```python
from build123d import *

# Parameters (mm, degrees)
SKETCH1_R             = 30
BOSS_EXTRUDE1_DEPTH   = 150
BOSS_EXTRUDE1_2_DEPTH = 150
EXTRUDE_THIN1_START   = -100
EXTRUDE_THIN1_DEPTH   = 100
SKETCH2_OUTSIDE_W     = 2224.156
SKETCH2_OUTSIDE_H     = 474.106
CUT_EXTRUDE1_DEPTH    = 100


# Read off the part's stored shape, not the designer's step: Extrude-Thin1
with BuildPart() as part:
    # Sketch1 → Boss-Extrude1 (new body)
    with BuildSketch(Plane(origin=(0, 0, 0), x_dir=(1, 0, 0), z_dir=(0, 1, 0))):
        with Locations(Location((0, 0, 0), (0, 0, 270))):
            Circle(SKETCH1_R)
    extrude(amount=-BOSS_EXTRUDE1_DEPTH)



with BuildPart() as body_2:
    # Sketch1 → Boss-Extrude1 2 (new body)
    with BuildSketch(Plane(origin=(0, 0, 0), x_dir=(1, 0, 0), z_dir=(0, 1, 0))):
        with Locations(Location((-1750.05, 0, 0), (0, 0, 270))):
            Circle(SKETCH1_R)
    extrude(amount=-BOSS_EXTRUDE1_2_DEPTH)


with BuildPart() as part_1:
    add(part.part)

    add(body_2.part)  # Extrude-Thin1 merges body 2
    # Extrude-Thin1 outline → Extrude-Thin1 (add)
    with BuildSketch(Plane.XY.offset(50).offset(EXTRUDE_THIN1_START)):
        with BuildLine():
            Line((-1500.05, -100), (-250, -100))
            add(Edge.make_bspline(
                [(-250, -100), (-180.532615563, -100), (-147.140452079, 0), (-100, 0)],
                knots=[0, 0, 0, 0, 1, 1, 1, 1], degree=3))
            Line((-100, 0), (50, 0))
            Line((50, 0), (50, 20))
            Line((50, 20), (-100, 20))
            add(Edge.make_bspline(
                [(-250, -80), (-246.8578922, -80), (-243.858737849, -79.72033393), (-237.993194947, -78.665321149), (-235.125426927, -77.888401959), (-229.419387385, -75.849767547), (-226.581615187, -74.586589055), (-220.900676803, -71.586264248), (-218.058608228, -69.848756808), (-212.373173985, -65.939898134), (-209.530533574, -63.76882272), (-203.856954109, -59.061240354), (-201.026304365, -56.525095932), (-195.383615818, -51.172709385), (-192.571647436, -48.356724406), (-186.962589328, -42.537122759), (-184.165515953, -39.533655599), (-178.571130319, -33.432647215), (-175.773867523, -30.335180457), (-170.151907521, -24.137576717), (-167.327345009, -21.037442901), (-161.608940626, -14.922554595), (-158.715354463, -11.907662629), (-152.79666366, -6.049585507), (-149.771886809, -3.205896979), (-143.499030151, 2.216662309), (-140.250865349, 4.796857765), (-133.403484489, 9.567046655), (-129.801981816, 11.759226892), (-124.033745357, 14.595891945), (-122.050123128, 15.465210164), (-117.953666514, 17.012030347), (-115.8406028, 17.689372637), (-111.491874555, 18.806547682), (-109.256121065, 19.246044187), (-104.688584729, 19.842959809), (-102.357022604, 20), (-100, 20)],
                knots=[0, 0, 0, 0, 0.0625, 0.0625, 0.125, 0.125, 0.1875, 0.1875, 0.25, 0.25, 0.3125, 0.3125, 0.375, 0.375, 0.4375, 0.4375, 0.5, 0.5, 0.5625, 0.5625, 0.625, 0.625, 0.6875, 0.6875, 0.75, 0.75, 0.8125, 0.8125, 0.875, 0.875, 0.90625, 0.90625, 0.9375, 0.9375, 0.96875, 0.96875, 1, 1, 1, 1], degree=3))
            Line((-250, -80), (-1500.05, -80))
            add(Edge.make_bspline(
                [(-1650.05, 20), (-1647.692977396, 20), (-1645.361415271, 19.842959809), (-1640.793878935, 19.246044187), (-1638.558125445, 18.806547682), (-1634.2093972, 17.689372637), (-1632.096333486, 17.012030347), (-1627.999876872, 15.465210164), (-1626.016254643, 14.595891945), (-1620.248018184, 11.759226892), (-1616.646515511, 9.567046655), (-1609.799134651, 4.796857765), (-1606.550969849, 2.216662309), (-1600.278113191, -3.205896979), (-1597.25333634, -6.049585507), (-1591.334645537, -11.907662629), (-1588.441059374, -14.922554595), (-1582.722654991, -21.037442901), (-1579.898092479, -24.137576717), (-1574.276132477, -30.335180457), (-1571.478869681, -33.432647215), (-1565.884484047, -39.533655599), (-1563.087410672, -42.537122759), (-1557.478352564, -48.356724406), (-1554.666384182, -51.172709385), (-1549.023695635, -56.525095932), (-1546.193045891, -59.061240354), (-1540.519466426, -63.76882272), (-1537.676826015, -65.939898134), (-1531.991391772, -69.848756808), (-1529.149323197, -71.586264248), (-1523.468384813, -74.586589055), (-1520.630612615, -75.849767547), (-1514.924573073, -77.888401959), (-1512.056805053, -78.665321149), (-1506.191262151, -79.72033393), (-1503.1921078, -80), (-1500.05, -80)],
                knots=[0, 0, 0, 0, 0.03125, 0.03125, 0.0625, 0.0625, 0.09375, 0.09375, 0.125, 0.125, 0.1875, 0.1875, 0.25, 0.25, 0.3125, 0.3125, 0.375, 0.375, 0.4375, 0.4375, 0.5, 0.5, 0.5625, 0.5625, 0.625, 0.625, 0.6875, 0.6875, 0.75, 0.75, 0.8125, 0.8125, 0.875, 0.875, 0.9375, 0.9375, 1, 1, 1, 1], degree=3))
            Line((-1650.05, 20), (-1800.05, 20))
            Line((-1800.05, 20), (-1800.05, 0))
            Line((-1800.05, 0), (-1650.05, 0))
            add(Edge.make_bspline(
                [(-1650.05, 0), (-1602.909547921, 0), (-1569.517384437, -100), (-1500.05, -100)],
                knots=[0, 0, 0, 0, 1, 1, 1, 1], degree=3))
        make_face()
    extrude(amount=EXTRUDE_THIN1_DEPTH)

    # Sketch2 outside → Cut-Extrude1 (cut)
    with BuildSketch(Plane(origin=(0, 0, 0), x_dir=(1, 0, 0), z_dir=(0, 1, 0))):
        with Locations((-875.025, 0)):
            Rectangle(SKETCH2_OUTSIDE_W, SKETCH2_OUTSIDE_H)
        with BuildLine():
            Line((0, -50), (-1750.05, -50))
            ThreePointArc((-1750.05, -50), (-1800.05, 0), (-1750.05, 50))
            Line((-1750.05, 50), (0, 50))
            ThreePointArc((0, 50), (50, 0), (0, -50))
        make_face(mode=Mode.SUBTRACT)
    extrude(amount=CUT_EXTRUDE1_DEPTH, mode=Mode.SUBTRACT)


solid = part_1.part
```
CAD build for the part. Positions are in the model's coordinates, mm. A direction names the side the tool comes from. Coordinates: 2 decimals unless noted, no trailing zeros. Order: outer loops, then holes, each group sorted by start corner. A loop starts at its lowest first (then second) coordinate and runs counter-clockwise, first axis right, second up. Notation, with made-up numbers: (72.25, 35.25) -> (92.25, 35.25) arc R6 ccw to (92.25, 45.25) -> close; hole circle Ø5 at (-23, 10.25). An arc over 180 degrees is marked (long way). Use one line per item in the form item = value. Start each with the question number.
1) Pull direction X, two halves, no side cores. Call faces 1 (the flat face through (-879, -89, -50)), 2 (the cylindrical face through (-1800.038, 9.86, 1.099)), 3 (the flat face through (-884, -100, -1)): +X half, -X half, draft (parallel to the pull), parting line (faces both ways), or undercut.
2) Drill centre lines: L1, parallel to X at y = -12.5, z = 11; L2, parallel to X at y = -29, z = 16; L3, parallel to Y at x = -1660.5, z = -15. Where is each one in solid material? Low to high. Write a range as [from, to].
3) Band-saw the part on B-B on x = -811. Give the cut face in (y, z).
4) Tool access for faces 4 (the cylindrical face through (49.988, 9.86, -1.099)), 5 (the flat face through (-866, -80, -1)), 6 (the cylindrical face through (1.32, -73.95, -29.97)): list every direction of +Z, -Z, +X, -X, +Y, -Y with a clear straight run to the whole face (end or side of a thin tool).
5) Band-saw the part on A-A on y = -60.5. State how many separate pieces and enclosed holes the cut face has, then the cut area to 3 significant figures.
6) Drop flat-ended pins along their axis: pin 1 (4 mm diameter, centred on x = -724.5, z = -12.5, fed in from -Y); pin 2 (1.5 mm diameter, centred on x = -478, z = -24.5, fed in from +Y); pin 3 (1.5 mm diameter, centred on x = -1115, y = -77.5, fed in from -Z). Give the stop position or say it passes through.
Entries:
q1.face_1 = draft
q1.face_2 = -X half
q1.face_3 = undercut
q2.L1 = [-1777.96, -1722.14], [-1620.26, -1590.8], [-159.25, -129.79], [-27.91, 27.91]
q2.L2 = [-1775.43, -1724.67], [-1602.68, -1575.49], [-174.56, -147.37], [-25.38, 25.38]
q2.L3 = [0, 20]
q3.outline = (-100, -50) -> (-80, -50) -> (-80, 50) -> (-100, 50) -> close
q4.face_4 = +X, +Y, -Y
q4.face_5 = +Z, -Z, +Y
q4.face_6 = -Y
q5.separate_pieces = 4
q5.enclosed_holes = 0
q5.area = 11,500 mm2
q6.pin_1 = -100
q6.pin_2 = -80
q6.pin_3 = through
